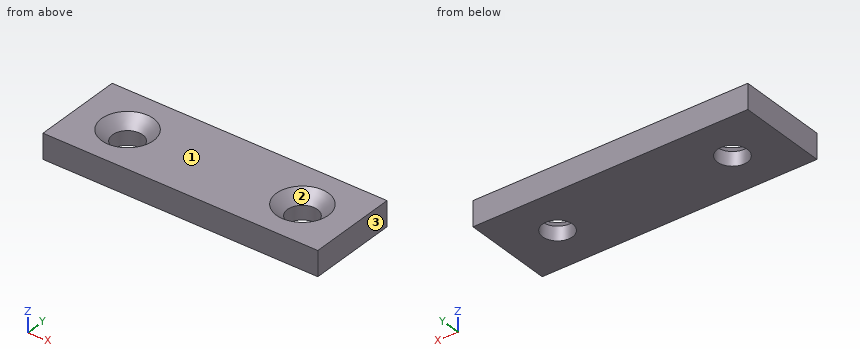
```python
from build123d import *

# Parameters (mm, degrees)
SKETCH2_W                      = 55
SKETCH2_H                      = 18
BOSS_EXTRUDE1_DEPTH            = 2.5
F_6_0MM_DOWEL_HOLE1_AT_2_COUNT = 2
F_6_0MM_DOWEL_HOLE1_AT_2_PITCH = 35


with BuildPart() as part:
    # Sketch2 → Boss-Extrude1 (new body, symmetric)
    with BuildSketch(Plane.XY):
        with Locations((27.5, 9)):
            Rectangle(SKETCH2_W, SKETCH2_H)
    extrude(amount=BOSS_EXTRUDE1_DEPTH, both=True)

    # Sketch3 → Ø6.0mm Dowel Hole1 (revolve, cut)
    with BuildSketch(Plane(origin=(10, 9, 2.5), x_dir=(0, -1, 0), z_dir=(1, 0, 0))):
        Polygon((0, 0), (0, 5), (3, 5), (3, 2.2), (5.2, 0), align=None)
    f_6_0mm_dowel_hole1 = revolve(axis=Axis((10, 9, 8.85), (0, 0, -1)), mode=Mode.SUBTRACT)

    # Ø6.0mm Dowel Hole1 at 2: Ø6.0mm Dowel Hole1 ×2
    with Locations(*[(i * F_6_0MM_DOWEL_HOLE1_AT_2_PITCH, 0, 0) for i in range(1, F_6_0MM_DOWEL_HOLE1_AT_2_COUNT)]):
        add(f_6_0mm_dowel_hole1, mode=Mode.SUBTRACT)


solid = part.part
```
Design review of the part built by this model. Coordinates are the model's own, in mm. Face numbers are marked on the shaded views. Give positions to 0.01 mm unless a question says otherwise; leave off trailing zeros. Order: outer loops, then holes, each group sorted by start corner. A loop starts at its lowest first (then second) coordinate and runs counter-clockwise, first axis right, second up. Notation, with made-up numbers: (19, 57.25) -> (30, 57.25) arc R9 cw to (30, 64.25) -> close; hole circle Ø7 at (-29.75, 28). An arc over 180 degrees is marked (long way). Write item = value, one per line. Start each with the question number.
(1) We need section A-A on y = 9. Write out the cut boundary in (x, z).
(2) For pin 1 (8 mm diameter, centred on x = 45, y = 9, fed in from +Z); pin 2 (3.5 mm diameter, centred on x = 10, y = 9, fed in from -Z), all flat-tipped, find the tip position at first contact; note any pin that passes through.
(3) We need section C-C on z = 1.35. Write out the cut boundary in (x, y).
(4) To check wall thickness, follow line 1 along X through (y, z) = (9, -1.75); line 2 along Y through (x, z) = (10, -1.2); line 3 along X through (y, z) = (6.5, 1.75). State the ranges of each line that lie inside material, in increasing order.
(5) We need section D-D on z = -1.35. Write out the cut boundary in (x, y), plus the area to 3 significant figures.
(6) We need section B-B on x = 10. Write out the cut boundary in (y, z), plus the area to 3 significant figures.
(7) Mouldability with a two-part tool opening along X and no side actions: class the marked faces 1, 2 and 3 as +X half, -X half, draft (parallel to the pull), parting line (faces both ways), or undercut.
Numbers:
q1.outline = (0, -2.5) -> (7, -2.5) -> (7, 0.3) -> (4.8, 2.5) -> (0, 2.5) -> close; (13, -2.5) -> (42, -2.5) -> (42, 0.3) -> (39.8, 2.5) -> (15.2, 2.5) -> (13, 0.3) -> close; (48, -2.5) -> (55, -2.5) -> (55, 2.5) -> (50.2, 2.5) -> (48, 0.3) -> close
q2.pin_1 = 1.3
q2.pin_2 = through
q3.outline = (0, 0) -> (55, 0) -> (55, 18) -> (0, 18) -> close; hole circle Ø8.1 at (10, 9); hole circle Ø8.1 at (45, 9)
q4.line_1 = 0 to 7, 13 to 42, 48 to 55
q4.line_2 = 0 to 6, 12 to 18
q4.line_3 = 0 to 6.32, 13.68 to 41.32, 48.68 to 55
q5.outline = (0, 0) -> (55, 0) -> (55, 18) -> (0, 18) -> close; hole circle Ø6 at (10, 9); hole circle Ø6 at (45, 9)
q5.area = 933 mm^2
q6.outline = (0, -2.5) -> (6, -2.5) -> (6, 0.3) -> (3.8, 2.5) -> (0, 2.5) -> close; (12, -2.5) -> (18, -2.5) -> (18, 2.5) -> (14.2, 2.5) -> (12, 0.3) -> close
q6.area = 55.2 mm^2
q7.face_1 = draft
q7.face_2 = undercut
q7.face_3 = +X half
